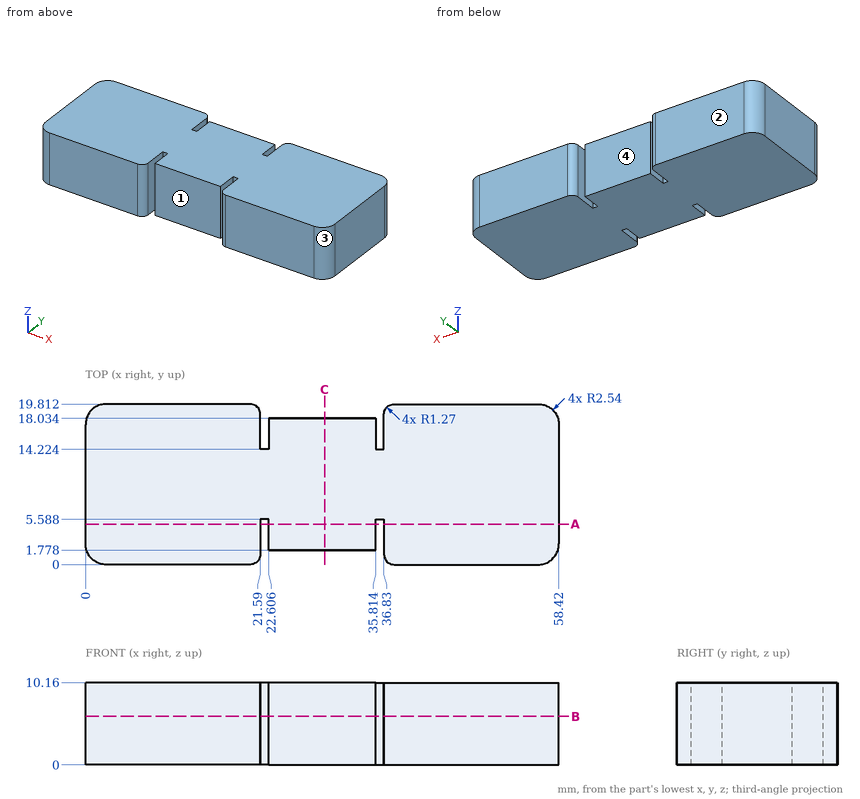
Can you work these out from the drawing? Everything is in mm from the part's minimum corner. Round coordinates to 2 decimals unless told otherwise and drop trailing zeros. Loops run counter-clockwise (first coordinate to the right, second up) from the corner with the lowest first, then second, coordinate; pieces in that order, holes last. Notation, with made-up numbers: (53, 11) - (85, 11) arc R30 ccw to (85, 38) - close; hole circle Ø2 at (26, 77.25). An arc over 180 degrees is marked (long way). Answer in a Markdown table with one row per item. Add a question column.
Q1. I want a section at A-A on y = 5. List the corners of the cut face in (x, z) for me.
Q2. I want a section at C-C on x = 29.5. List the corners of the cut face in (y, z) for me.
Q3. We'd pull the mould along X, two halves only. Please class the marked faces 1, 2, 3 and 4: pulls with the +X half, pulls with the -X half, needs draft (parallel to the pull), parting line crosses it, or undercut.
Q4. For pin 1 Ø3 at (x, z) = (30, 4.5) entering from -Y; pin 2 Ø1.1 at (x, z) = (36.5, 6) entering from +Y; pin 3 Ø2 at (x, z) = (35, 2) entering from +Y, each with a flat end and sliding along its axis, tell me the tip position at first contact or that it passes through.
Q5. I want a section at B-B on z = 6. List the corners of the cut face in (x, y) for me.
Q6. I need wall thicknesses on L1, parallel to X at y = 2.75, z = 7; L2, parallel to Y at x = 33, z = 3.75; L3, parallel to X at y = 19, z = 1.5. Which ranges of each line are inside material? Lowest first, please.
A:
| question | item | result |
|---|---|---|
| 1 | outline | (0, 0) - (21.59, 0) - (21.59, 10.16) - (0, 10.16) - close; (22.61, 0) - (35.81, 0) - (35.81, 10.16) - (22.61, 10.16) - close; (36.83, 0) - (58.42, 0) - (58.42, 10.16) - (36.83, 10.16) - close |
| 2 | outline | (1.78, 0) - (18.03, 0) - (18.03, 10.16) - (1.78, 10.16) - close |
| 3 | face 1 | undercut |
| 3 | face 2 | needs draft |
| 3 | face 3 | pulls with the +X half |
| 3 | face 4 | undercut |
| 4 | pin 1 | y = 1.78 |
| 4 | pin 2 | y = 19.26 |
| 4 | pin 3 | y = 18.03 |
| 5 | outline | (0, 2.54) arc R2.54 ccw to (2.54, 0) - (20.32, 0) arc R1.27 ccw to (21.59, 1.27) - (21.59, 5.59) - (22.61, 5.59) - (22.61, 1.78) - (35.81, 1.78) - (35.81, 5.59) - (36.83, 5.59) - (36.83, 1.27) arc R1.27 ccw to (38.1, 0) - (55.88, 0) arc R2.54 ccw to (58.42, 2.54) - (58.42, 17.27) arc R2.54 ccw to (55.88, 19.81) - (38.1, 19.81) arc R1.27 ccw to (36.83, 18.54) - (36.83, 14.22) - (35.81, 14.22) - (35.81, 18.03) - (22.61, 18.03) - (22.61, 14.22) - (21.59, 14.22) - (21.59, 18.54) arc R1.27 ccw to (20.32, 19.81) - (2.54, 19.81) arc R2.54 ccw to (0, 17.27) - close |
| 6 | L1 | 0 to 21.59, 22.61 to 35.81, 36.83 to 58.42 |
| 6 | L2 | 1.78 to 18.03 |
| 6 | L3 | 0.68 to 21.5, 36.92 to 57.74 |
